Work out the finished part from the listing and answer in its coordinate system (mm). Face numbers are marked on the shaded views. Coordinates: 2 decimals unless noted, no trailing zeros. Order: outer loops, then holes, each group sorted by start corner. A loop starts at its lowest first (then second) coordinate and runs counter-clockwise, first axis right, second up. Notation, with made-up numbers: (82, -31) -> (109, -31) arc R17 cw to (109, 1) -> close; hole circle Ø1 at (61.5, 47). An arc over 180 degrees is marked (long way). Write item = value, one per line. Start each with the question number.
Q1. The part is cut by section A-A, the plane y = 0. Determine the outline of the cut face in (x, z) (3 decimals), plus the area to 4 significant figures.
Q2. Straight lines are drawn through the part: L1, parallel to Y at x = 1.15, z = 2; L2, parallel to Y at x = 0.5, z = 4.75; L3, parallel to X at y = -1.2, z = 5 (3 decimals). For each, find the intervals that lie inside material, in ascending order. Write a range as from..to.
Q3. For a pull along X with two mould halves and no side action, classify the marked faces 1, 2, 3 and 4 as +X half, -X half, draft (parallel to the pull), parting line (faces both ways), or undercut.
Q4. The part is cut by section C-C, the plane x = -0.35. Determine the outline of the cut face in (y, z), plus the area to 3 significant figures.
Q5. The part is cut by section B-B, the plane z = 2.25. Determine the outline of the cut face in (x, y) (3 decimals), plus the area to 3 significant figures.
Q6. Flat-ended cylindrical pins translate along their axes: pin 1 (2.5 mm diameter, centred on x = 1.5, y = -0.5, fed in from +Z); pin 2 (2 mm diameter, centred on x = 2, y = -2, fed in from -Z). Find the tip coordinate at first contact, or state that the pin passes through.
Q7. The part is cut by section D-D, the plane y = 1.6. Determine the outline of the cut face in (x, z) (3 decimals), plus the area to 3 significant figures.
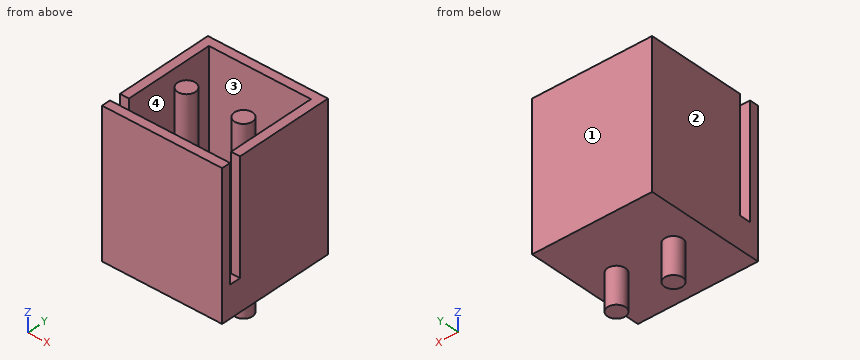
```python
from build123d import *

# Parameters (mm, degrees)
SKETCH_1_W          = 5.35
SKETCH_1_H          = 5.3
EXTRUDE_1_DEPTH     = 6.4
SKETCH_2_W          = 4.55
SKETCH_2_H          = 4.5
SKETCH_2_R          = 0.4
CUT_EXTRUDE_1_DEPTH = 5
SKETCH_3_W          = 12.899416502
SKETCH_3_H          = 0.501475964
CUT_EXTRUDE_2_DEPTH = 5
SKETCH_4_R          = 0.4
EXTRUDE_2_DEPTH     = 8


with BuildPart() as part:
    # Эскиз1 → Вытянуть1 (new body)
    with BuildSketch(Plane.XY):
        Rectangle(SKETCH_1_W, SKETCH_1_H)
    extrude(amount=EXTRUDE_1_DEPTH)

    # Эскиз2 → Вырез-Вытянуть1 (cut)
    with BuildSketch(Plane.XY.offset(6.4)):
        Rectangle(SKETCH_2_W, SKETCH_2_H)
        with Locations((-1.27, 0)):
            Circle(SKETCH_2_R, mode=Mode.SUBTRACT)
        with Locations((1.27, 0)):
            Circle(SKETCH_2_R, mode=Mode.SUBTRACT)
    extrude(amount=-CUT_EXTRUDE_1_DEPTH, mode=Mode.SUBTRACT)

    # Эскиз3 → Вырез-Вытянуть2 (cut)
    with BuildSketch(Plane.XY.offset(6.4)):
        with Locations((-0.066925705, -2.002104797)):
            Rectangle(SKETCH_3_W, SKETCH_3_H)
    extrude(amount=-CUT_EXTRUDE_2_DEPTH, mode=Mode.SUBTRACT)

    # Эскиз4 → Вытянуть2 (add)
    with BuildSketch(Plane.XY.offset(6.4)):
        with Locations((-1.27, 0)):
            Circle(SKETCH_4_R)
        with Locations((1.27, 0)):
            Circle(SKETCH_4_R)
    extrude(amount=-EXTRUDE_2_DEPTH)


solid = part.part
```
Model answer:
q1.outline = (-2.675, 0) -> (-1.67, 0) -> (-1.67, -1.6) -> (-0.87, -1.6) -> (-0.87, 0) -> (0.87, 0) -> (0.87, -1.6) -> (1.67, -1.6) -> (1.67, 0) -> (2.675, 0) -> (2.675, 6.4) -> (2.275, 6.4) -> (2.275, 1.4) -> (1.67, 1.4) -> (1.67, 6.4) -> (0.87, 6.4) -> (0.87, 1.4) -> (-0.87, 1.4) -> (-0.87, 6.4) -> (-1.67, 6.4) -> (-1.67, 1.4) -> (-2.275, 1.4) -> (-2.275, 6.4) -> (-2.675, 6.4) -> close
q1.area = 22.05 mm2
q2.L1 = -2.65..-2.25, -0.38..0.38, 2.25..2.65
q2.L2 = -2.65..-2.25, 2.25..2.65
q2.L3 = -2.675..-2.275, 2.275..2.675
q3.face_1 = draft
q3.face_2 = -X half
q3.face_3 = undercut
q3.face_4 = undercut
q4.outline = (-2.65, 0) -> (2.65, 0) -> (2.65, 6.4) -> (2.25, 6.4) -> (2.25, 1.4) -> (-2.25, 1.4) -> (-2.25, 6.4) -> (-2.65, 6.4) -> close
q4.area = 11.4 mm2
q5.outline = (-2.675, -2.65) -> (2.675, -2.65) -> (2.675, -2.253) -> (-2.675, -2.253) -> close; (-2.675, -1.751) -> (-2.275, -1.751) -> (-2.275, 2.25) -> (2.275, 2.25) -> (2.275, -1.751) -> (2.675, -1.751) -> (2.675, 2.65) -> (-2.675, 2.65) -> close; circle Ø0.8 at (-1.27, 0); circle Ø0.8 at (1.27, 0)
q5.area = 8.47 mm2
q6.pin_1 = 6.4
q6.pin_2 = 0
q7.outline = (-2.675, 0) -> (2.675, 0) -> (2.675, 6.4) -> (2.275, 6.4) -> (2.275, 1.4) -> (-2.275, 1.4) -> (-2.275, 6.4) -> (-2.675, 6.4) -> close
q7.area = 11.5 mm2
